Design review of the part built by this model. Coordinates are the model's own, in mm. Coordinates: 2 decimals unless noted, no trailing zeros. Write each loop counter-clockwise with the first axis right and the second up, starting at its lowest first coordinate (ties: lowest second). Pieces come first, ordered by that corner, then holes.
Q1. For pin 1 Ø7.5 at (x, y) = (56.36, 63.5) entering from -Z; pin 2 Ø8 at (x, z) = (208, 12.5) entering from +Y, all flat-tipped, find the tip position at first contact; note any pin that passes through.
Q2. For L1, parallel to X at y = 628, z = 12.75; L2, parallel to X at y = 893.5, z = 1.75; L3, parallel to Y at x = 168.5, z = 17, list the stretches that pass through material, from the lowest coordinate up.
Q3. Take a section at B-B, the plane y = 775.5. Write out the cut boundary in (x, z), plus the area to 3 significant figures.
Q4. Take a section at A-A, the plane z = 3.75. Write out the cut boundary in (x, y).
Q5. Take a section at C-C, the plane x = 339. Write out the cut boundary in (y, z).
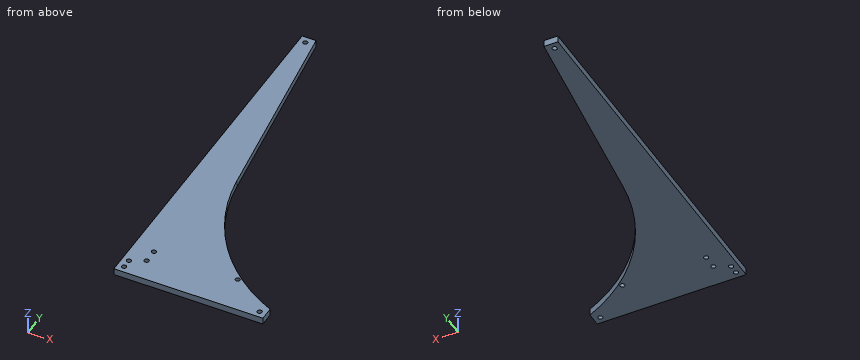
from build123d import *

# Parameters (mm, degrees)
SKETCH1_R           = 6.35
BOSS_EXTRUDE1_DEPTH = 18.25625


with BuildPart() as part:
    # Sketch1 → Boss-Extrude1 (new body)
    with BuildSketch(Plane.XY):
        with BuildLine():
            Line((0, 0), (406.4, 0))
            Line((406.4, 0), (406.4, 38.1))
            ThreePointArc((406.4, 38.1), (207.539140749, 196.40002074), (111.667415652, 431.8))
            Line((111.667415652, 431.8), (38.1, 990.6))
            Line((38.1, 990.6), (0, 990.6))
            Line((0, 990.6), (0, 0))
        make_face()
        with Locations((18.25625, 18.25625)):
            Circle(SKETCH1_R, mode=Mode.SUBTRACT)
        with Locations((388.14375, 18.25625)):
            Circle(SKETCH1_R, mode=Mode.SUBTRACT)
        with Locations((18.25625, 972.34375)):
            Circle(SKETCH1_R, mode=Mode.SUBTRACT)
        with Locations((56.35625, 101.6)):
            Circle(SKETCH1_R, mode=Mode.SUBTRACT)
        with Locations((284.95625, 101.6)):
            Circle(SKETCH1_R, mode=Mode.SUBTRACT)
        with Locations((18.25625, 43.65625)):
            Circle(SKETCH1_R, mode=Mode.SUBTRACT)
        with Locations((56.35625, 63.5)):
            Circle(SKETCH1_R, mode=Mode.SUBTRACT)
    extrude(amount=BOSS_EXTRUDE1_DEPTH)


solid = part.part
Responses:
1. pin 1: passes through
1. pin 2: stops at y = 201.19
2. L1: x = 0 to 85.84
2. L2: x = 0 to 50.88
2. L3: y = 0 to 257.23
3. outline: (0, 0) - (66.42, 0) - (66.42, 18.26) - (0, 18.26) - close
3. area: 1,210 mm2
4. outline: (0, 0) - (406.4, 0) - (406.4, 38.1) arc R502.17 cw to (111.67, 431.8) - (38.1, 990.6) - (0, 990.6) - close; hole circle Ø12.7 at (18.26, 18.26); hole circle Ø12.7 at (18.26, 43.66); hole circle Ø12.7 at (18.26, 972.34); hole circle Ø12.7 at (56.36, 63.5); hole circle Ø12.7 at (56.36, 101.6); hole circle Ø12.7 at (284.96, 101.6); hole circle Ø12.7 at (388.14, 18.26)
5. outline: (0, 0) - (74.28, 0) - (74.28, 18.26) - (0, 18.26) - close
